Input: part model. Units: mm. Frame: model coordinates. A direction names the side the tool comes from. Coordinates: 2 decimals unless noted, no trailing zeros. Write each loop counter-clockwise with the first axis right and the second up, starting at its lowest first coordinate (ties: lowest second). Pieces come first, ordered by that corner, then holes.
from build123d import *

# Parameters (mm, degrees)
BOSS_EXTRUDE1_DEPTH = 107.75
SKETCH2_W           = 8.5
SKETCH2_H           = 5
BOSS_EXTRUDE2_DEPTH = 4.25
SKETCH3_W           = 8.5
SKETCH3_H           = 2.5
CUT_EXTRUDE1_DEPTH  = 3.25
SKETCH4_W           = 1.75
SKETCH4_H           = 2.5
BOSS_EXTRUDE3_DEPTH = 4.75
SKETCH5_W           = 1.75
SKETCH5_H           = 2.5
BOSS_EXTRUDE4_DEPTH = 4.75
SKETCH7_W           = 121.985175889
SKETCH7_H           = 106.89742867
CUT_EXTRUDE4_DEPTH  = 4.5


with BuildPart() as part:
    # Sketch1 → Boss-Extrude1 (new body)
    with BuildSketch(Plane.XY):
        Polygon((-61.3, -24.208957416), (-61.3, -22.458957416), (-67.8, -22.458957416), (-67.8, -31.208957416), (67.8, -31.208957416), (67.8, -22.458957416), (61.3, -22.458957416), (61.3, -24.208957416), (66.05, -24.208957416), (66.05, -26.708957416), (-66.05, -26.708957416), (-66.05, -24.208957416), align=None)
    extrude(amount=-BOSS_EXTRUDE1_DEPTH)

    # Sketch2 → Boss-Extrude2 (add)
    with BuildSketch(Plane(origin=(0, -26.708957416, 0), x_dir=(1, 0, 0), z_dir=(0, 1, 0))):
        with Locations((-13.5, 105.25)):
            Rectangle(SKETCH2_W, SKETCH2_H)
        with Locations((35.3, 105.25)):
            Rectangle(SKETCH2_W, SKETCH2_H)
    extrude(amount=BOSS_EXTRUDE2_DEPTH)

    # Sketch3 → Cut-Extrude1 (cut)
    with BuildSketch(Plane.XY.offset(-102.75)):
        with Locations((-13.5, -25.458957416)):
            Rectangle(SKETCH3_W, SKETCH3_H)
        with Locations((35.3, -25.458957416)):
            Rectangle(SKETCH3_W, SKETCH3_H)
    extrude(amount=-CUT_EXTRUDE1_DEPTH, mode=Mode.SUBTRACT)

    # Sketch4 → Boss-Extrude3 (add)
    with BuildSketch(Plane.ZY.offset(-66.05)):
        with Locations((-106.875, -25.458957416)):
            Rectangle(SKETCH4_W, SKETCH4_H)
    extrude(amount=BOSS_EXTRUDE3_DEPTH)

    # Sketch5 → Boss-Extrude4 (add)
    with BuildSketch(Plane(origin=(-66.05, 0, 0), x_dir=(0, 0, -1), z_dir=(1, 0, 0))):
        with Locations((106.875, -25.458957416)):
            Rectangle(SKETCH5_W, SKETCH5_H)
    extrude(amount=BOSS_EXTRUDE4_DEPTH)

    # Sketch7 → Cut-Extrude4 (cut)
    with BuildSketch(Plane.XZ.offset(31.208957416)):
        with Locations((-1.007412056, -49.301285665)):
            Rectangle(SKETCH7_W, SKETCH7_H)
    extrude(amount=-CUT_EXTRUDE4_DEPTH, mode=Mode.SUBTRACT)


solid = part.part
Item 1: Material intervals for line 1 (X direction, y = -23.75, z = -59); line 2 (X direction, y = -25, z = -62.5); line 3 (Z direction, x = 48, y = -29.75), sorted ascending.
Item 2: Pull-direction query (Y, two-part tool) for faces 1 (the face through (-17.75, -24, -106)), 2 (the face through (-65, -22.459, -53)), 3 (the face through (-14, -24.209, -104)); classes: released by +Y, released by -Y, zero draft, split by the parting line, or undercut.
Item 3: Section query B-B, the plane y = -28.5. Return loops of the section in (x, z).
Item 4: Section query A-A, the plane z = -63. Return loops of the section in (x, y).
Item 5: Section query C-C, the plane x = -31.5. Return loops of the section in (y, z), then the cut area to 3 significant figures.
Item 6: Pin query (flat end, axial travel): pin 1 Ø1.9 at (x, y) = (-14.5, -23) entering from +Z; pin 2 Ø1.2 at (x, y) = (-62.5, -25.5) entering from +Z. Return the tip coordinate at first contact, or that it passes through.
Item 7: Access query for faces 4 (the face through (-62, -29, -52)), 5 (the face through (-2, -29, -102.75)), 6 (the face through (61.3, -23, -55)). Directions: +Z, -Z, +X, -X, +Y, -Y. A direction counts if a zero-diameter tool reaches every point of the face in a straight line with its end or side. Return the directions, or none.
The answers:
1. line 1: x = -67.8 to -61.3, 61.3 to 67.8
1. line 2: x = -67.8 to -66.05, 66.05 to 67.8
1. line 3: z = -107.75 to -102.75
2. face 1: zero draft
2. face 2: released by +Y
2. face 3: undercut
3. outline: (-67.8, -107.75) - (67.8, -107.75) - (67.8, 0) - (59.99, 0) - (59.99, -102.75) - (-62, -102.75) - (-62, 0) - (-67.8, 0) - close
4. outline: (-67.8, -31.21) - (-62, -31.21) - (-62, -26.71) - (-66.05, -26.71) - (-66.05, -24.21) - (-61.3, -24.21) - (-61.3, -22.46) - (-67.8, -22.46) - close; (59.99, -31.21) - (67.8, -31.21) - (67.8, -22.46) - (61.3, -22.46) - (61.3, -24.21) - (66.05, -24.21) - (66.05, -26.71) - (59.99, -26.71) - close
5. outline: (-31.21, -107.75) - (-26.71, -107.75) - (-26.71, -102.75) - (-31.21, -102.75) - close
5. area: 22.5 mm2
6. pin 1: stops at z = -102.75
6. pin 2: stops at z = -106
7. face 4: +Z, -Y
7. face 5: +Z, +Y, -Y
7. face 6: +Z, -Z, +Y
